```python
from build123d import *

# Parameters (mm, degrees)
BOSS_EXTRUDE1_DEPTH = 76.2
SHELL1_T            = -2.54
CUT_EXTRUDE1_DEPTH  = 2.54
CIRPATTERN1_COUNT   = 4


with BuildPart() as part:
    # Sketch1 → Boss-Extrude1 (new body)
    with BuildSketch(Plane(origin=(0, 0, 0), x_dir=(1, 0, 0), z_dir=(0, 1, 0))):
        Polygon((0, 0), (0, -41.892312512), (-63.5, -41.892312512), (-63.5, 16.822913885), (-16.822913885, 63.5), (76.2, 63.5), (76.2, 0), align=None)
    extrude(amount=BOSS_EXTRUDE1_DEPTH)

    # Shell1
    shell1_openings = [part.faces().sort_by_distance(p)[0] for p in [
        (-31.75, 38.1, 41.892312512),
    ]]
    offset(amount=SHELL1_T, openings=shell1_openings, kind=Kind.INTERSECTION)

    # Sketch4 → Cut-Extrude1 (cut)
    with BuildSketch(Plane(origin=(76.2, 0, 0), x_dir=(0, 0, -1), z_dir=(1, 0, 0))):
        with BuildLine():
            Line((29.845, 46.228), (33.655, 46.228))
            ThreePointArc((33.655, 46.228), (35.433, 44.45), (33.655, 42.672))
            Line((33.655, 42.672), (29.845, 42.672))
            ThreePointArc((29.845, 42.672), (28.067, 44.45), (29.845, 46.228))
        make_face()
    cut_extrude1 = extrude(amount=-CUT_EXTRUDE1_DEPTH, mode=Mode.SUBTRACT)

    # CirPattern1: Cut-Extrude1 ×4 about axis
    cirpattern1_axis = Axis((0, 38.1, -31.75), (1, 0, 0))
    for i in range(1, CIRPATTERN1_COUNT):
        add(cut_extrude1.rotate(cirpattern1_axis, i * 360 / CIRPATTERN1_COUNT), mode=Mode.SUBTRACT)


solid = part.part
```
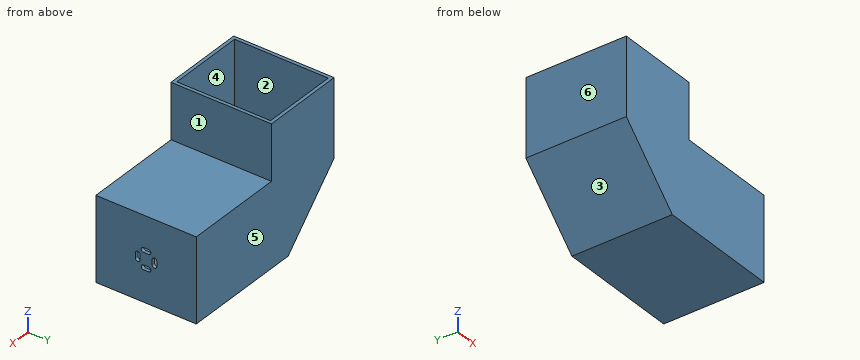
Check sheet for the modelled part. Datum: model origin and axes. Units: mm. Face numbers are marked on the shaded views. A direction names the side the tool comes from. Give positions to 0.01 mm unless a question says otherwise; leave off trailing zeros. Loops run counter-clockwise (first coordinate to the right, second up) from the corner with the lowest first, then second, coordinate; pieces in that order, holes last. Notation, with made-up numbers: M 69,50.5 L 99,50.5 A16 ccw 99,72.5 Z; hole C -22,-34 d6. An arc over 180 degrees is marked long. Answer as CSV lines item,"result".
Item 1: Set-up check for the marked faces 1, 2 and 3: record each of +Z, -Z, +X, -X, +Y, -Y from which the full face is reachable in a straight line by a thin tool's end or side.
Reply:
face 1,"+Z, +X, +Y, -Y"
face 2,"+Z"
face 3,"-Z, -X, +Y, -Y"
Item 2: Scan lines: L1, parallel to Y at x = -26, z = 29.5; L2, parallel to Z at x = 6, y = 35. Record each from-to range of solid material in increasing order.
Reply:
L1,"0 to 2.54, 73.66 to 76.2"
L2,"-63.5 to -60.96, -2.54 to 0"
Item 3: Sectioned sample at D-D, the plane x = -13. Enter the section's corners in (y, z), then the cut area to 3 significant figures.
Reply:
outline,"M 0,-63.5 L 76.2,-63.5 L 76.2,41.89 L 73.66,41.89 L 73.66,-60.96 L 2.54,-60.96 L 2.54,41.89 L 0,41.89 Z"
area,"716 mm^2"
Item 4: Sectioned sample at A-A, the plane x = 25. Enter the section's corners in (y, z).
Reply:
outline,"M 0,-63.5 L 76.2,-63.5 L 76.2,0 L 0,0 Z; hole M 2.54,-60.96 L 73.66,-60.96 L 73.66,-2.54 L 2.54,-2.54 Z"
Item 5: Sectioned sample at C-C, the plane z = 35. Enter the section's corners in (x, y), then the cut area to 3 significant figures.
Reply:
outline,"M -63.5,0 L 0,0 L 0,76.2 L -63.5,76.2 Z; hole M -60.96,2.54 L -2.54,2.54 L -2.54,73.66 L -60.96,73.66 Z"
area,"684 mm^2"
Item 6: Sectioned sample at B-B, the plane y = 44.45. Enter the section's corners in (x, z).
Reply:
outline,"M -63.5,-16.82 L -16.82,-63.5 L 76.2,-63.5 L 76.2,-35.43 L 73.66,-35.43 L 73.66,-60.96 L -15.77,-60.96 L -60.96,-15.77 L -60.96,41.89 L -63.5,41.89 Z; M -2.54,-2.54 L 73.66,-2.54 L 73.66,-28.07 L 76.2,-28.07 L 76.2,0 L 0,0 L 0,41.89 L -2.54,41.89 Z"
Item 7: Draft check along X on the marked faces 4, 5 and 6. Enter one of: pulls with the +X half, pulls with the -X half, needs draft (parallel to the pull), parting line crosses it, or undercut.
Reply:
face 4,"undercut"
face 5,"needs draft"
face 6,"pulls with the -X half"
Item 8: Depth check by flat-ended pin: pin 1 Ø21.5 at (x, y) = (46, 51) entering from +Z; pin 2 Ø1 at (y, z) = (46.5, -20.5) entering from -X; pin 3 Ø12.5 at (y, z) = (26, 22) entering from +X. Enter the tip coordinate at first touch or a pass-through.
Reply:
pin 1,"z = 0"
pin 2,"x = -60.32"
pin 3,"x = 0"
